Source: CAD feature listing. Evaluate the final solid. Frame: model axes, mm. A direction names the side the tool comes from. Round coordinates to 2 decimals unless told otherwise and drop trailing zeros. Loops run counter-clockwise (first coordinate to the right, second up) from the corner with the lowest first, then second, coordinate; pieces in that order, holes last.
Item 1: Pull-direction query (Y, two-part tool) for faces 5 (the flat face through (26.8, 16, 4)), 6 (the cylindrical face through (26.087, -5.748, 4.409)), 7 (the cylindrical face through (26.394, 16.559, 10.498)); classes: released by +Y, released by -Y, zero draft, split by the parting line, or undercut.
Item 2: Access query for faces 1 (the flat face through (-0.5, 24, 1)), 2 (the flat face through (26.4, 23, 1)), 3 (the cylindrical face through (-0.76, 16.559, 10.498)), 4 (the flat face through (5, 5.25, -1)). Directions: +Z, -Z, +X, -X, +Y, -Y. A direction counts if a zero-diameter tool reaches every point of the face in a straight line with its end or side. Return the directions, or none.
Item 3: Section query B-B on y = 13.5. Return loops of the section in (x, z).
Item 4: Ray query, L1, parallel to Y at x = 1, z = -1.45; L2, parallel to X at y = 35, z = -0.9; L3, parallel to X at y = 2.5, z = 6.25. Return the intervals inside material, ascending.
Item 5: Section query C-C on z = 5.5. Return loops of the section in (x, y).
Item 6: Section query D-D on z = 10. Return loops of the section in (x, y).
Item 7: First-contact query: P1, Ø6, axis at y = 23.5, z = 2.5, coming from the -X side; P2, Ø1.5, axis at y = 3.5, z = 2, coming from the -X side; P3, Ø6, axis at x = 22, y = 24.5, coming from the +Z side; P4, Ø2.5, axis at y = 2.5, z = 3.5, coming from the +X side. Flat tips, straight axial feed; report the tip coordinate or a pass-through.
```python
from build123d import *
from build123d.topology import SkipClean

# Parameters (mm, degrees)
SKETCH_1_R          = 1.1
SKETCH_1_W          = 26
SKETCH_1_H          = 32.5
EXTRUDE_1_DEPTH     = 11
EXTRUDE_START       = 2
SKETCH_3_R          = 1.1
EXTRUDE_2_DEPTH     = 2
SKETCH_2_R          = 1.1
CUT_EXTRUDE_1_DEPTH = 49.250803102
SKETCH_4_W          = 8
SKETCH_4_H          = 15
CUT_EXTRUDE_3_DEPTH = 10
SKETCH_5_R          = 6.5
CUT_EXTRUDE_4_DEPTH = 49.250803102
FILLET_START        = -2
FILLET_1_DEPTH      = 30
SKETCH_6_R          = 2.5
CUT_EXTRUDE_5_DEPTH = 0.4
CUT_EXTRUDE_START   = -1
SKETCH_7_R          = 2.5
CUT_EXTRUDE_6_DEPTH = 1


with BuildPart() as part:
    # ｽｹｯﾁ1 → ﾎﾞｽ - 押し出し1 (new body)
    with BuildSketch(Plane.XY):
        with BuildLine():
            Line((26.8, 35), (26.8, -4))
            ThreePointArc((26.8, -4), (26.067766953, -5.767766953), (24.3, -6.5))
            Line((24.3, -6.5), (1, -6.5))
            ThreePointArc((1, -6.5), (-0.767766953, -5.767766953), (-1.5, -4))
            Line((-1.5, -4), (-1.5, 35))
            ThreePointArc((-1.5, 35), (-0.767766953, 36.767766953), (1, 37.5))
            Line((1, 37.5), (24.3, 37.5))
            ThreePointArc((24.3, 37.5), (26.067766953, 36.767766953), (26.8, 35))
        make_face()
        with Locations((21.8, 35)):
            Circle(SKETCH_1_R, mode=Mode.SUBTRACT)
        with Locations((1, 35)):
            Circle(SKETCH_1_R, mode=Mode.SUBTRACT)
        with Locations((1, -4)):
            Circle(SKETCH_1_R, mode=Mode.SUBTRACT)
        with Locations((21.8, -4)):
            Circle(SKETCH_1_R, mode=Mode.SUBTRACT)
        with Locations((13, 16.25)):
            Rectangle(SKETCH_1_W, SKETCH_1_H, mode=Mode.SUBTRACT)
    extrude(amount=EXTRUDE_1_DEPTH)

    # ｽｹｯﾁ3 → ﾎﾞｽ - 押し出し2 (add)
    with SkipClean():  # the faces are left unmerged after this step: merging them gives an invalid solid
        with BuildSketch(Plane(origin=(0, 0, 0), x_dir=(-1, 0, 0), z_dir=(0, 0, -1)).offset(EXTRUDE_START)):
            with BuildLine():
                Line((1.5, -4), (1.5, 35))
                ThreePointArc((1.5, 35), (0.767766953, 36.767766953), (-1, 37.5))
                Line((-1, 37.5), (-24.3, 37.5))
                ThreePointArc((-24.3, 37.5), (-26.067766953, 36.767766953), (-26.8, 35))
                Line((-26.8, 35), (-26.8, -4))
                ThreePointArc((-26.8, -4), (-26.067766953, -5.767766953), (-24.3, -6.5))
                Line((-24.3, -6.5), (-1, -6.5))
                ThreePointArc((-1, -6.5), (0.767766953, -5.767766953), (1.5, -4))
            make_face()
            with Locations((-21.8, -4)):
                Circle(SKETCH_3_R, mode=Mode.SUBTRACT)
            with Locations((-1, -4)):
                Circle(SKETCH_3_R, mode=Mode.SUBTRACT)
            with Locations((-1, 35)):
                Circle(SKETCH_3_R, mode=Mode.SUBTRACT)
            with Locations((-21.8, 35)):
                Circle(SKETCH_3_R, mode=Mode.SUBTRACT)
        extrude(amount=-EXTRUDE_2_DEPTH)

    # ｽｹｯﾁ2 → ｶｯﾄ - 押し出し1 (cut, through all)
    with SkipClean():  # the faces are left unmerged after this step: merging them gives an invalid solid
        with BuildSketch(Plane.ZY.offset(1.5)):
            with Locations(Location((2.5, 23.5, 0), (0, 0, 270))):
                Circle(SKETCH_2_R)
            with Locations(Location((2.5, 2.5, 0), (0, 0, 270))):
                Circle(SKETCH_2_R)
        extrude(amount=-CUT_EXTRUDE_1_DEPTH, mode=Mode.SUBTRACT)

    # ｽｹｯﾁ4 → ｶｯﾄ - 押し出し3 (cut)
    with SkipClean():  # the faces are left unmerged after this step: merging them gives an invalid solid
        with BuildSketch(Plane(origin=(0, 0, -2), x_dir=(-1, 0, 0), z_dir=(0, 0, -1))):
            with Locations((-5.25, 12.75)):
                Rectangle(SKETCH_4_W, SKETCH_4_H)
        extrude(amount=-CUT_EXTRUDE_3_DEPTH, mode=Mode.SUBTRACT)

    # ｽｹｯﾁ5 → ｶｯﾄ - 押し出し4 (cut, through all)
    with SkipClean():  # the faces are left unmerged after this step: merging them gives an invalid solid
        with BuildSketch(Plane(origin=(26.8, 0, 0), x_dir=(0, 0, -1), z_dir=(1, 0, 0))):
            with Locations((-13, 23.5)):
                Circle(SKETCH_5_R)
        extrude(amount=-CUT_EXTRUDE_4_DEPTH, mode=Mode.SUBTRACT)

    # ﾌｨﾚｯﾄ1: read off the stored shape, not the designer's step
    # ﾌｨﾚｯﾄ1 outline → ﾌｨﾚｯﾄ1 (cut)
    with SkipClean():  # the faces are left unmerged after this step: merging them gives an invalid solid
        with BuildSketch(Plane.YZ.offset(FILLET_START)):
            with BuildLine():
                ThreePointArc((14.375856205, 11), (16.587485547, 10.484272031), (18.342875246, 9.043478261))
                ThreePointArc((18.342875246, 9.043478261), (17.745349201, 9.977750147), (17.315341562, 11))
                Line((17.315341562, 11), (14.375856205, 11))
            make_face()
            with BuildLine():
                ThreePointArc((29.684658438, 11), (29.254650799, 9.977750147), (28.657124754, 9.043478261))
                ThreePointArc((28.657124754, 9.043478261), (30.412514453, 10.484272031), (32.624143795, 11))
                Line((32.624143795, 11), (29.684658438, 11))
            make_face()
        extrude(amount=FILLET_1_DEPTH, mode=Mode.SUBTRACT)

    # ｽｹｯﾁ6 → ｶｯﾄ - 押し出し5 (cut)
    with SkipClean():  # the faces are left unmerged after this step: merging them gives an invalid solid
        with BuildSketch(Plane(origin=(26.8, 0, 0), x_dir=(0, 0, -1), z_dir=(1, 0, 0))):
            with Locations((-2.5, 2.5)):
                Circle(SKETCH_6_R)
            with Locations((-2.5, 23.5)):
                Circle(SKETCH_6_R)
        extrude(amount=-CUT_EXTRUDE_5_DEPTH, mode=Mode.SUBTRACT)

    # ｽｹｯﾁ7 → ｶｯﾄ - 押し出し6 (cut)
    with SkipClean():  # the faces are left unmerged after this step: merging them gives an invalid solid
        with BuildSketch(Plane.ZY.offset(1.5).offset(CUT_EXTRUDE_START)):
            with Locations(Location((2.5, 2.5, 0), (0, 0, 180))):
                Circle(SKETCH_7_R)
            with Locations(Location((2.5, 23.5, 0), (0, 0, 180))):
                Circle(SKETCH_7_R)
        extrude(amount=CUT_EXTRUDE_6_DEPTH, mode=Mode.SUBTRACT)


solid = part.part
```
Data:
1. face 5: zero draft
1. face 6: released by -Y
1. face 7: undercut
2. face 1: -X
2. face 2: +X
2. face 3: +Z, +X, -X
2. face 4: +Z, -Z
3. outline: (-1.5, -2) - (1.25, -2) - (1.25, 0) - (0, 0) - (0, 11) - (-1.5, 11) - close; (9.25, -2) - (26.8, -2) - (26.8, 11) - (26, 11) - (26, 0) - (9.25, 0) - close
4. L1: y = -6.5 to -5.1, -2.9 to 33.9, 36.1 to 37.5
4. L2: x = -1.5 to -0.1, 2.1 to 20.7, 22.9 to 26.8
4. L3: x = -1.5 to 0, 26 to 26.8
5. outline: (-1.5, -4) arc R2.5 ccw to (1, -6.5) - (24.3, -6.5) arc R2.5 ccw to (26.8, -4) - (26.8, 35) arc R2.5 ccw to (24.3, 37.5) - (1, 37.5) arc R2.5 ccw to (-1.5, 35) - close; hole circle Ø2.2 at (1, -4); hole circle Ø2.2 at (1, 35); hole (0, 0) - (26, 0) - (26, 32.5) - (0, 32.5) - close; hole circle Ø2.2 at (21.8, -4); hole circle Ø2.2 at (21.8, 35)
6. outline: (-1.5, -4) arc R2.5 ccw to (1, -6.5) - (24.3, -6.5) arc R2.5 ccw to (26.8, -4) - (26.8, 17.38) - (26, 17.38) - (26, 0) - (0, 0) - (0, 17.38) - (-1.5, 17.38) - close; (-1.5, 29.62) - (0, 29.62) - (0, 32.5) - (26, 32.5) - (26, 29.62) - (26.8, 29.62) - (26.8, 35) arc R2.5 ccw to (24.3, 37.5) - (1, 37.5) arc R2.5 ccw to (-1.5, 35) - close; hole circle Ø2.2 at (1, -4); hole circle Ø2.2 at (1, 35); hole circle Ø2.2 at (21.8, -4); hole circle Ø2.2 at (21.8, 35)
7. P1: stops at x = -1.5
7. P2: stops at x = -0.5
7. P3: stops at z = 0
7. P4: stops at x = 26.4
